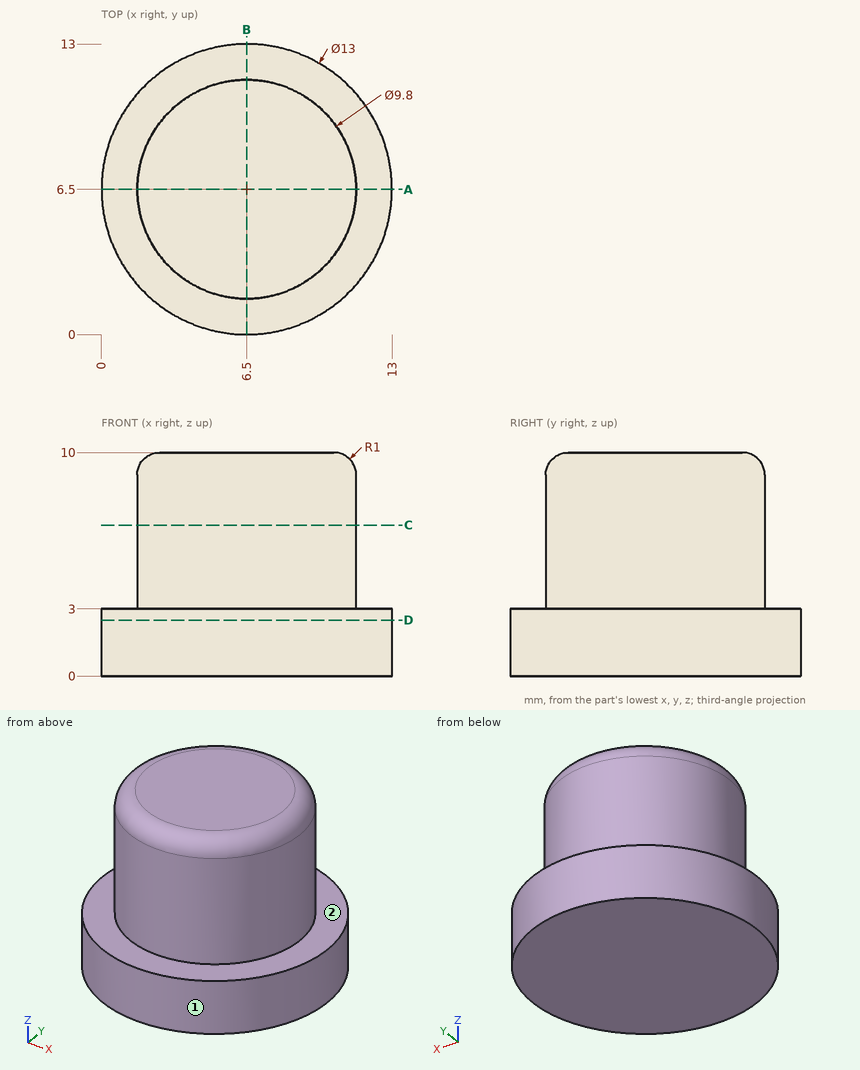
The drawing under review shows one solid part. Ordinate dimensions are in mm from its lowest x, y, z. A direction names the side the tool comes from. Coordinates: 2 decimals unless noted, no trailing zeros. Write each loop counter-clockwise with the first axis right and the second up, starting at its lowest first coordinate (ties: lowest second). Pieces come first, ordered by that corner, then holes. Notation, with made-up numbers: (27.5, 25.25) -> (80.5, 25.25) arc R18 cw to (80.5, 40.25) -> close; hole circle Ø5 at (-25.75, 65.5). An arc over 180 degrees is marked (long way). Write each question's results on one line, items separated by ' | '. Start each with the question number.
1) Insertion check: pin 1 (1.5 mm diameter, centred on x = 10, z = 5, fed in from -Y); pin 2 (5 mm diameter, centred on x = 4.5, z = 6.5, fed in from -Y); pin 3 (1 mm diameter, centred on y = 11.5, z = 6, fed in from +X). Each pin has a flat end and moves straight along its axis. Give the tip position at first contact, or say it passes through.
2) Wall thickness on L1, parallel to Z at x = 11.25, y = 4.5; L2, parallel to X at y = 9, z = 4.75; L3, parallel to Y at x = 8.25, z = 6.25: over which ranges is each line inside the solid? List them lowest first. Write a range as [from, to].
3) Consider section D-D (z = 2.5). Write out the cut boundary in (x, y), plus the area to 3 significant figures.
4) Consider section A-A (y = 6.5). Write out the cut boundary in (x, z), plus the area to 3 significant figures.
5) Consider section C-C (z = 6.75). Write out the cut boundary in (x, y).
6) For the marked faces 1 and 2, list the 3-axis set-ups (+Z, -Z, +X, -X, +Y, -Y) from which the entire face can be reached by the end or side of a thin tool; tool diameter is ignored.
Geometry says:
1) pin 1: y = 2.44 | pin 2: y = 1.6 | pin 3: x = 8.44
2) L1: [0, 3] | L2: [2.29, 10.71] | L3: [1.92, 11.08]
3) outline: circle Ø13 at (6.5, 6.5) | area: 133 mm^2
4) outline: (0, 0) -> (13, 0) -> (13, 3) -> (11.4, 3) -> (11.4, 9) arc R1 ccw to (10.4, 10) -> (2.6, 10) arc R1 ccw to (1.6, 9) -> (1.6, 3) -> (0, 3) -> close | area: 107 mm^2
5) outline: circle Ø9.8 at (6.5, 6.5)
6) face 1: +Z, -Z | face 2: +Z
